CAD build for the part. Positions are in the model's coordinates, mm. Give positions to 0.01 mm unless a question says otherwise; leave off trailing zeros. Write each loop counter-clockwise with the first axis right and the second up, starting at its lowest first coordinate (ties: lowest second). Pieces come first, ordered by that corner, then holes. Notation, with made-up numbers: (-3.5, -9.5) - (0.5, -9.5) arc R27 ccw to (0.5, 27.5) - close; hole circle Ø5 at (0, 31.25). An arc over 180 degrees is marked (long way). Answer as a JSON object with one key per item and string values.
Autodesk Inventor part; units mm, degrees
ref_plane "YZ Plane" through (0, 0, 0) normal (1, 0, 0) x (0, 1, 0)
ref_plane "XZ Plane" through (0, 0, 0) normal (0, 1, 0) x (-1, 0, 0)
ref_plane "XY Plane" through (0, 0, 0) normal (0, 0, 1) x (1, 0, 0)
sketch "Sketch1" plane through (0, 0, 0) normal (0, 1, 0) x (-1, 0, 0)
  line L0 (0, 0) -> (15, 0)
  line L1 (15, 0) -> (15, -30)
  line L2 (15, -30) -> (0, -30)
  line L3 (0, -30) -> (0, 0)
  line L4 (7.5, 0) -> (7.5, -157.6812)
  line L5 (7.5, 0) -> (165.1812, 0) construction
  line L6 (7.5, -157.6812) -> (7.5, -150.1812)
  circle A0 centre (7.5, -150.1812) radius 7.5
  circle A1 centre (7.5, -7.5) radius 7.5
  circle A2 centre (7.5, -22.5) radius 7.5
  circle A3 centre (7.5, -7.5) radius 2.75
  line L7 (15, 0) -> (0, 0)
  line L8 (0, 0) -> (0, -157.6812)
  line L9 (0, -157.6812) -> (15, -157.6812)
  line L10 (15, -157.6812) -> (15, 0)
  circle A4 centre (7.5, -150.1812) radius 2.75
  circle A5 centre (7.5, -22.5) radius 2.75
  point P0 (0, -150.1812)
  point P1 (15, -150.1812)
  point P2 (15, -7.5)
  point P3 (0, -7.5)
  point P4 (7.5, -15)
  dimension "d9" = 15
  dimension "d10" = 30
  dimension "d11" = 157.6812
  dimension "d12" = 90
  dimension "d13" = 7.5
  dimension "d14" = 15
  dimension "d15" = 15
  dimension "d16" = 15
  dimension "d17" = 5.5
  dimension "d18" = 5.5
  dimension "d19" = 5.5
extrude "Extrusion1" add sketch "Sketch1" along normal blind 2 contours A1 L4 A3 | L4 A3 A1 | A1 A2 L3 | L1 A2 A1 | A2 L2 L3 | A2 L4 A5 | A2 L4 A5 | L1 L2 A2 | L2 L4 A0 L8 | L2 L10 A0 L4 | A0 L4 A4 | A0 L4 A4
extrude "Extrusion2" add sketch "Sketch1" along normal blind 3 contours A1 L4 A3 | L4 A3 A1 | A2 L4 A5 | A2 L4 A5
extrude "Extrusion3" cut sketch "Sketch1" along normal mid plane 2 contours A3 L4 | L4 A3 | A5 L4 | L4 A5 | A4 L4 | L4 A4
extrude "Extrusion4" add sketch "Sketch1" along normal blind 4 contours A1 L4 A3 | L4 A3 A1 | A2 L4 A5 | A2 L4 A5
properties part number "közeplsoszalag1"
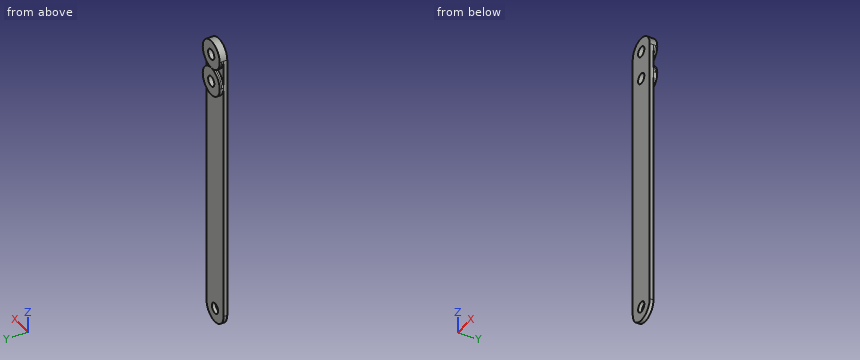
Item 1: Cut at C-C (x = -13). Give the cut face in (y, z).
Entries:
{"outline": "(0, -155.28) - (2, -155.28) - (2, -27.6) - (4, -27.6) - (4, -17.4) - (2, -17.4) - (2, -12.6) - (4, -12.6) - (4, -2.4) - (0, -2.4) - close"}
Item 2: Probe line 1 (Z direction, x = -7.5, y = 1.8); line 2 (Z direction, x = -9, y = 0.25); line 3 (X direction, y = 1.5, z = -22.5). List the from-to ranges inside material, lowest first. Write a range as from..to.
Entries:
{"line 1": "-157.68..-152.93, -147.43..-25.25, -19.75..-10.25, -4.75..0", "line 2": "-157.53..-152.49, -147.88..-24.8, -20.2..-9.8, -5.2..-0.15", "line 3": "-15..-10.25, -4.75..0"}
Item 3: Cut at A-A (y = 1.4). Give the cut face in (x, z).
Entries:
{"outline": "(-15, -150.18) arc R7.5 ccw to (0, -150.18) - (0, -7.5) arc R7.5 ccw to (-15, -7.5) - close; hole circle Ø5.5 at (-7.5, -150.18); hole circle Ø5.5 at (-7.5, -22.5); hole circle Ø5.5 at (-7.5, -7.5)"}
Item 4: Cut at D-D (x = -3.25). Give the cut face in (y, z), and give its area (3 significant figures).
Entries:
{"outline": "(0, -156.36) - (2, -156.36) - (2, -28.68) - (4, -28.68) - (4, -16.32) - (2, -16.32) - (2, -13.68) - (4, -13.68) - (4, -1.32) - (0, -1.32) - close", "area": "360 mm2"}
Item 5: Flat gauge pins, fed straight in: P1, Ø1, axis at x = -12.5, y = 0.5, coming from the +Z side; P2, Ø5, axis at x = -7.5, z = -150.18, coming from the +Y side; P3, Ø1, axis at x = -11.5, y = 3.5, coming from the +Z side. Where does each tip first touch, or does it go through?
Entries:
{"P1": "z = -1.5", "P2": "through", "P3": "z = -0.87"}
Item 6: Cut at B-B (z = -64.5). Give the cut face in (x, y).
Entries:
{"outline": "(-15, 0) - (0, 0) - (0, 2) - (-15, 2) - close"}
